Check sheet for the modelled part. Datum: model origin and axes. Units: mm. A direction names the side the tool comes from. Round coordinates to 2 decimals unless told otherwise and drop trailing zeros. Loops run counter-clockwise (first coordinate to the right, second up) from the corner with the lowest first, then second, coordinate; pieces in that order, holes last. Notation, with made-up numbers: (20, -33) -> (65, -33) arc R20 cw to (65, 5) -> close; hole circle Ø10 at (63, -39.5). An arc over 180 degrees is marked (long way). Use one line per item in the form item = value. Start each with the question number.
(1) Set-up check for faces 5 (the flat face through (-1, 1, 0)), 6 (the flat face through (15, 10, 5)), 7 (the flat face through (-15, 10, 5)), 8 (the flat face through (0, 2, 5)), 9 (the flat face through (19, 5, 5)): record each of +Z, -Z, +X, -X, +Y, -Y from which the full face is reachable in a straight line by a thin tool's end or side.
(2) Draft check along Y on faces 1 (the flat face through (-13, 8, 5)), 2 (the cylindrical face through (0, 21, 5)), 3 (the flat face through (17, 5, 5)), 4 (the flat face through (0, 0, 5)). Enter one of: released by +Y, released by -Y, zero draft, split by the parting line, or undercut.
(3) Sectioned sample at C-C (x = 0). Record the cut outline in (y, z).
(4) Sectioned sample at A-A (y = 3.5). Record the cut outline in (x, z), and give its area (3 significant figures).
(5) Material ranges on probe 1 along Y at (x, z) = (13, 6); probe 2 along Y at (x, z) = (0, 2.5); probe 3 along X at (y, z) = (6.75, 1), recorded low to high. Write a range as [from, to].
(6) Sectioned sample at D-D (y = 19.5). Record the cut outline in (x, z), and give its area (3 significant figures).
(7) Go/stop test with flat-tipped pins: pin 1 (4 mm diameter, centred on x = -14, z = 5, fed in from +Y); pin 2 (1.5 mm diameter, centred on y = 17, z = 7, fed in from -X). Record where each tip stops, or that it passes through.
(8) Sectioned sample at B-B (z = 8.25). Record the cut outline in (x, y).
from build123d import *

# Parameters (mm, degrees)
EXTRUDE_THIN1_DEPTH = 10


with BuildPart() as part:
    # Sketch1 → Extrude-Thin1 (new body)
    with BuildSketch(Plane.XY):
        with BuildLine():
            Line((11, 10), (19, 10))
            Line((19, 10), (19, 0))
            Line((19, 0), (-19, 0))
            Line((-19, 0), (-19, 10))
            Line((-19, 10), (-11, 10))
            ThreePointArc((-11, 10), (0, 21), (11, 10))
        make_face()
        with BuildLine():
            Line((8.774964387, 8), (17, 8))
            Line((17, 8), (17, 2))
            Line((17, 2), (-17, 2))
            Line((-17, 2), (-17, 8))
            Line((-17, 8), (-8.774964387, 8))
            ThreePointArc((-8.774964387, 8), (0, 19), (8.774964387, 8))
        make_face(mode=Mode.SUBTRACT)
    extrude(amount=EXTRUDE_THIN1_DEPTH)


solid = part.part
Checks:
q1.face_5 = -Z, +X, -X, +Y, -Y
q1.face_6 = +Z, -Z, +X, +Y
q1.face_7 = +Z, -Z, -X, +Y
q1.face_8 = +Z, -Z
q1.face_9 = +Z, -Z, +X, +Y, -Y
q2.face_1 = undercut
q2.face_2 = released by +Y
q2.face_3 = undercut
q2.face_4 = released by -Y
q3.outline = (0, 0) -> (2, 0) -> (2, 10) -> (0, 10) -> close; (19, 0) -> (21, 0) -> (21, 10) -> (19, 10) -> close
q4.outline = (-19, 0) -> (-17, 0) -> (-17, 10) -> (-19, 10) -> close; (17, 0) -> (19, 0) -> (19, 10) -> (17, 10) -> close
q4.area = 40.0 mm2
q5.probe_1 = [0, 2], [8, 10]
q5.probe_2 = [0, 2], [19, 21]
q5.probe_3 = [-19, -17], [17, 19]
q6.outline = (-5.55, 0) -> (5.55, 0) -> (5.55, 10) -> (-5.55, 10) -> close
q6.area = 111 mm2
q7.pin_1 = 10
q7.pin_2 = -9.05
q8.outline = (-19, 0) -> (19, 0) -> (19, 10) -> (11, 10) arc R11 ccw to (-11, 10) -> (-19, 10) -> close; hole (-17, 2) -> (17, 2) -> (17, 8) -> (8.77, 8) arc R9 ccw (long way) to (-8.77, 8) -> (-17, 8) -> close
